For this review, take the finished solid that the model builds, in its own axes (mm). A direction names the side the tool comes from. Coordinates: 2 decimals unless noted, no trailing zeros. Answer as a JSON object with one key per item and string values. Group by question number.
1) Draft analysis for pull direction Z (two halves, no side actions). For faces 3 (the flat face through (-163, 8, 15.5)), 4 (the flat face through (-161.418, 13.2, -22.686)), 5 (the cylindrical face through (-156.4, 37.1, -0.3)), 6 (the flat face through (-184, 0, 0)), state which applies: +Z half, -Z half, draft (parallel to the pull), parting line (faces both ways), or undercut.
2) Machinability: for faces 1 (the conical face through (-171.6, 29.6, -0.3)), 2 (the flat face through (-163, 8, -15.5)), which of the approach directions +Z, -Z, +X, -X, +Y, -Y give a long, thin tool a straight path to every point of the face, cutting with its end or side? Answer none if there is none.
3) Wall thickness on L1, parallel to Z at x = -160.5, y = 15; L2, parallel to Z at x = -164.5, y = 18.5; L3, parallel to X at y = 10.5, z = -16: over which ranges is each line inside the solid? List them lowest first.
4) For pin 1 (2 mm diameter, centred on x = -183, z = -16.5, fed in from +Y); pin 2 (8 mm diameter, centred on x = -163, y = 50, fed in from +Z); pin 3 (4 mm diameter, centred on x = -182.5, z = 10, fed in from +Y), all flat-tipped, find the tip position at first contact; note any pin that passes through.
from build123d import *

# Parameters (mm, degrees)
REVOLVE1_ANGLE           = 8
REVOLVE1_OTHER_WAY_ANGLE = 8
CUT_EXTRUDE1_DEPTH       = 15.5
CUT_EXTRUDE1_DEPTH_BACK  = 15.5
FILLET1_R                = 6


with BuildPart() as part:
    # Sketch4 → Revolve1 (revolve)
    with BuildSketch(Plane.XY):
        Polygon((-156.4, 0), (-156.4, 60), (-186.4, 0), align=None)
    revolve(axis=Axis((0, 70, 0), (0, -1, 0)), revolution_arc=REVOLVE1_ANGLE)

    # Sketch4 → Revolve1 other way (revolve)
    with BuildSketch(Plane.XY):
        Polygon((-156.4, 0), (-156.4, 60), (-186.4, 0), align=None)
    revolve(axis=Axis((0, 70, 0), (0, 1, 0)), revolution_arc=REVOLVE1_OTHER_WAY_ANGLE)

    # Sketch6 → Cut-Extrude1 (cut, two sides: drawn at the far end of the back side and taken through both)
    with BuildSketch(Plane.XY.offset(-CUT_EXTRUDE1_DEPTH_BACK)):
        Polygon((-154.877925951, 28.284271247), (-183.162197199, 0), (-154.877925951, 0), align=None)
    extrude(amount=CUT_EXTRUDE1_DEPTH + CUT_EXTRUDE1_DEPTH_BACK, mode=Mode.SUBTRACT)

    # Fillet1
    fillet1_edges = [part.edges().sort_by_distance(p)[0] for p in [
        (-169.731946982, 30, 23.854269505),
        (-169.731946982, 30, -23.854269505),
    ]]
    fillet(fillet1_edges, radius=FILLET1_R)


solid = part.part
Output values:
{
 "1": {"face 3": "undercut", "face 4": "-Z half", "face 5": "undercut", "face 6": "draft"},
 "2": {"face 1": "-X, +Y", "face 2": "+X, -Y"},
 "3": {"L1": "z = -22.56 to -15.5, 15.5 to 22.56", "L2": "z = -23.12 to -15.5, 15.5 to 23.12", "L3": "x = -180.44 to -155.58"},
 "4": {"pin 1": "stops at y = 7.32", "pin 2": "stops at z = 20.17", "pin 3": "stops at y = 11.25"}
}
